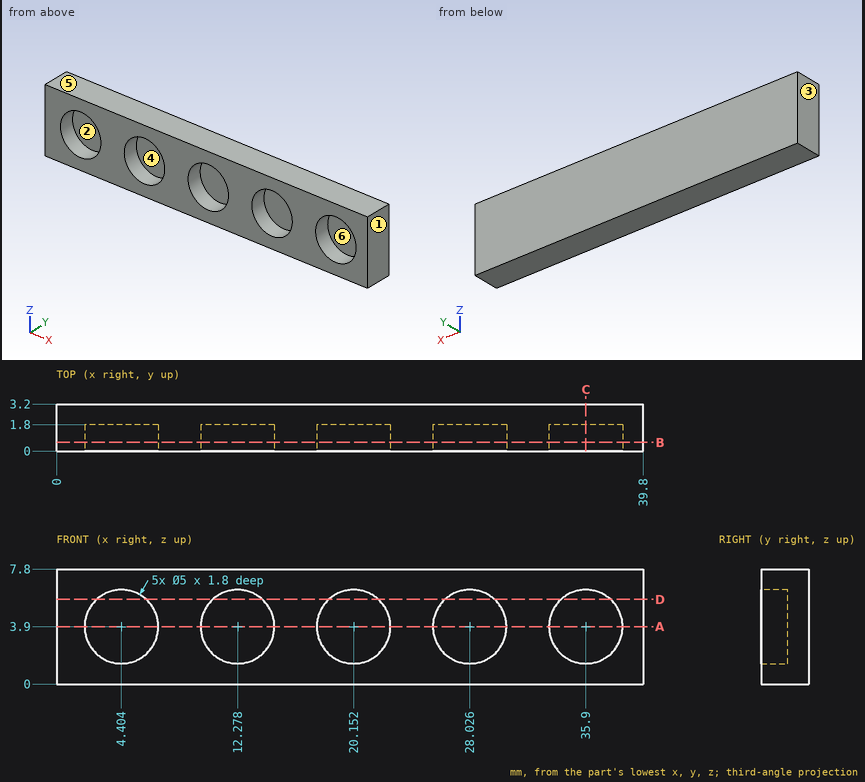
Verification items for this drawing (mm, ordinates from the low corner). A direction names the side the tool comes from. Coordinates: 2 decimals unless noted, no trailing zeros. Write each loop counter-clockwise with the first axis right and the second up, starting at its lowest first coordinate (ties: lowest second). Pieces come first, ordered by that corner, then holes. Notation, with made-up numbers: M 53.25,44 L 87.25,44 A23 cw 87.25,79 Z; hole C -35.5,42 d9. An arc over 180 degrees is marked long. One line per item, written item: value. Start each with the question number.
(1) Sectioned sample at D-D, the plane z = 5.75. Enter the section's corners in (x, y), and give its area (3 significant figures).
(2) Scan lines: line 1 along X through (y, z) = (0.45, 3.9); line 2 along Z through (x, y) = (36, 0.55); line 3 along X through (y, z) = (1.15, 5.5). Record each from-to range of solid material in increasing order. Write a range as [from, to].
(3) Sectioned sample at C-C, the plane x = 35.9. Enter the section's corners in (y, z), and give its area (3 significant figures).
(4) Sectioned sample at A-A, the plane z = 3.9. Enter the section's corners in (x, y).
(5) Depth check by flat-ended pin: pin 1 (4.5 mm diameter, centred on x = 4.404, z = 3.9, fed in from -Y). Enter the tip coordinate at first touch or a pass-through.
(6) Release check for a two-part mould opening along X. For the marked faces 1, 2, 3 and 4 record: released by +X, released by -X, zero draft, split by the parting line, or undercut.
(7) Sectioned sample at B-B, the plane y = 0.6. Enter the section's corners in (x, z).
(8) Tool access check on the marked faces 5 and 6. Record the directions out of +Z, -Z, +X, -X, +Y, -Y that give a thin tool (end or side, any length) a straight path to the whole face; none if there is none.
Filled sheet:
1. outline: M 0,0 L 2.72,0 L 2.72,1.8 L 6.09,1.8 L 6.09,0 L 10.6,0 L 10.6,1.8 L 13.96,1.8 L 13.96,0 L 18.47,0 L 18.47,1.8 L 21.83,1.8 L 21.83,0 L 26.34,0 L 26.34,1.8 L 29.71,1.8 L 29.71,0 L 34.22,0 L 34.22,1.8 L 37.58,1.8 L 37.58,0 L 39.8,0 L 39.8,3.2 L 0,3.2 Z
1. area: 97.1 mm²
2. line 1: [0, 1.9], [6.9, 9.78], [14.78, 17.65], [22.65, 25.53], [30.53, 33.4], [38.4, 39.8]
2. line 2: [0, 1.4], [6.4, 7.8]
2. line 3: [0, 2.48], [6.32, 10.36], [14.2, 18.23], [22.07, 26.11], [29.95, 33.98], [37.82, 39.8]
3. outline: M 0,0 L 3.2,0 L 3.2,7.8 L 0,7.8 L 0,6.4 L 1.8,6.4 L 1.8,1.4 L 0,1.4 Z
3. area: 16.0 mm²
4. outline: M 0,0 L 1.9,0 L 1.9,1.8 L 6.9,1.8 L 6.9,0 L 9.78,0 L 9.78,1.8 L 14.78,1.8 L 14.78,0 L 17.65,0 L 17.65,1.8 L 22.65,1.8 L 22.65,0 L 25.53,0 L 25.53,1.8 L 30.53,1.8 L 30.53,0 L 33.4,0 L 33.4,1.8 L 38.4,1.8 L 38.4,0 L 39.8,0 L 39.8,3.2 L 0,3.2 Z
5. pin 1: y = 1.8
6. face 1: released by +X
6. face 2: undercut
6. face 3: released by -X
6. face 4: undercut
7. outline: M 0,0 L 39.8,0 L 39.8,7.8 L 0,7.8 Z; hole C 4.4,3.9 d5; hole C 12.28,3.9 d5; hole C 20.15,3.9 d5; hole C 28.03,3.9 d5; hole C 35.9,3.9 d5
8. face 5: +Z, +X, -X, +Y, -Y
8. face 6: -Y
